Read the model definition and answer for the solid it produces. Units are mm, in the model's axes. A direction names the side the tool comes from. Give positions to 0.01 mm unless a question says otherwise; leave off trailing zeros. Order: outer loops, then holes, each group sorted by start corner. A loop starts at its lowest first (then second) coordinate and runs counter-clockwise, first axis right, second up. Notation, with made-up numbers: (-29, 85.5) - (-8, 85.5) arc R29 cw to (-8, 118.5) - close; hole circle Ø6 at (-37.75, 56.25). An arc over 180 degrees is marked (long way). Write item = value, one per line.
```python
from build123d import *

# Parameters (mm, degrees)
PAD005_DEPTH    = 10
SKETCH015_W     = 4
SKETCH015_H     = 1.5
SKETCH016_R     = 1.6
POCKET003_DEPTH = 10.061


with BuildPart() as part:
    # Sketch014 → Pad005 (new body)
    with BuildSketch(Plane.YZ):
        with BuildLine():
            Line((-17.5, 0), (-6.06, 0))
            ThreePointArc((6.06, 0), (0, 6.06), (-6.06, 0))
            Line((6.06, 0), (15, 0))
            Line((15, 0), (15, 6))
            Line((15, 6), (8.074875, 6))
            ThreePointArc((8.074875, 6), (0, 10.06), (-8.074875, 6))
            Line((-8.074875, 6), (-17.5, 6))
            Line((-17.5, 0), (-17.5, 6))
        make_face()
    extrude(amount=PAD005_DEPTH)

    # Sketch015 → Groove005 (revolve, cut)
    with BuildSketch(Plane.XY):
        with Locations((8, 6.81)):
            Rectangle(SKETCH015_W, SKETCH015_H)
        with Locations((2, 6.81)):
            Rectangle(SKETCH015_W, SKETCH015_H)
    revolve(axis=Axis((0, 0, 0), (1, 0, 0)), mode=Mode.SUBTRACT)

    # Sketch016 → Pocket003 (cut, through all)
    with BuildSketch(Plane.XY):
        with Locations((5, 11.537437)):
            Circle(SKETCH016_R)
        with Locations((5, -12.787437)):
            Circle(SKETCH016_R)
    extrude(amount=POCKET003_DEPTH, mode=Mode.SUBTRACT)


solid = part.part
```
1. For faces 4 (the face through (5, -11, 6)), 5 (the face through (4, 10, 6)), 6 (the face through (4, 0, 6.3)), determine the directions among +Z, -Z, +X, -X, +Y, -Y from which every point of the face is accessible in a straight line to the end or side of a thin tool.
Recorded:
face_4 = +Z, +X, -X, -Y
face_5 = +Z, +X, -X, +Y
face_6 = -Z, -X
2. Section A-A (x = 5) is taken. Determine the outline of the cut face in (y, z), and give its area (3 significant figures).
Recorded:
outline = (-17.5, 0) - (-14.39, 0) - (-14.39, 6) - (-17.5, 6) - close; (-11.19, 0) - (-6.06, 0) arc R6.06 cw to (6.06, 0) - (9.94, 0) - (9.94, 6) - (8.07, 6) arc R10.06 ccw to (-8.07, 6) - (-11.19, 6) - close; (13.14, 0) - (15, 0) - (15, 6) - (13.14, 6) - close
area = 145 mm^2
3. A flat-ended cylindrical pin translates along its axis: pin 1 (4.5 mm diameter, centred on x = 6.5, y = -14, fed in from +Z). Find the tip coordinate at first contact, or state that the pin passes through.
Recorded:
pin_1 = 6
4. Section C-C (y = 0) is taken. Determine the outline of the cut face in (x, z).
Recorded:
outline = (0, 7.56) - (4, 7.56) - (4, 6.06) - (6, 6.06) - (6, 7.56) - (10, 7.56) - (10, 10.06) - (0, 10.06) - close
5. Section B-B (x = 2.25) is taken. Determine the outline of the cut face in (y, z), and give its area (3 significant figures).
Recorded:
outline = (-17.5, 0) - (-7.56, 0) arc R7.56 cw to (7.56, 0) - (15, 0) - (15, 6) - (8.07, 6) arc R10.06 ccw to (-8.07, 6) - (-17.5, 6) - close
area = 151 mm^2
6. Straight lines are drawn through the part: L1, parallel to Y at x = 5, z = 3.9; L2, parallel to Y at x = 5, z = 3.4; L3, parallel to Z at x = 4.75, y = -9. For each, find the intervals that lie inside material, in ascending order. Write a range as [from, to].
Recorded:
L1 = [-17.5, -14.39], [-11.19, -4.64], [4.64, 9.94], [13.14, 15]
L2 = [-17.5, -14.39], [-11.19, -5.02], [5.02, 9.94], [13.14, 15]
L3 = [0, 6]
7. Determine the mould class of faces 1 (the face through (4.65, -14.35, 2.96)), 2 (the face through (6, 0, 6.3)), 3 (the face through (8.03, 0.17, 7.56)) for opening direction X: +X half, -X half, draft (parallel to the pull), parting line (faces both ways), or undercut.
Recorded:
face_1 = undercut
face_2 = +X half
face_3 = draft
8. Section D-D (z = 8) is taken. Determine the outline of the cut face in (x, y), and give its area (3 significant figures).
Recorded:
outline = (0, -6.1) - (10, -6.1) - (10, 6.1) - (0, 6.1) - close
area = 122 mm^2
